Autodesk Inventor part; units mm, degrees
ref_plane "YZ Plane" through (0, 0, 0) normal (1, 0, 0) x (0, 1, 0)
ref_plane "XZ Plane" through (0, 0, 0) normal (0, 1, 0) x (-1, 0, 0)
ref_plane "XY Plane" through (0, 0, 0) normal (0, 0, 1) x (1, 0, 0)
sketch "スケッチ1" plane through (0, 0, 0) normal (0, 1, 0) x (-1, 0, 0)
  circle A0 centre (0, 0) radius 4 construction
  line L0 (0, 0) -> (0, -4.9846) construction
  line L1 (0, 0) -> (4.0815, -2.3565) construction
  line L2 (3.4641, -2) -> (0, -4)
  line L3 (3.4641, 2) -> (3.4641, -2)
  line L4 (0, 4) -> (3.4641, 2)
  line L5 (-3.4641, 2) -> (0, 4)
  line L6 (-3.4641, -2) -> (-3.4641, 2)
  line L7 (0, -4) -> (-3.4641, -2)
  dimension "d0" = 8
  dimension "d1" = 60
  dimension "d4" = 360
extrude "押し出し1" add sketch "スケッチ1" along normal blind 3
fillet "フィレット1" radius 0.5 6 edges at (1.7321, 3, 3) (-1.7321, 3, 3) (-3.4641, 3, 0) (-1.7321, 3, -3) (1.7321, 3, -3) (3.4641, 3, 0)
fillet "フィレット2" radius 0.1 6 edges at (1.7321, 0, 3) (-1.7321, 0, 3) (-3.4641, 0, 0) (-1.7321, 0, -3) (1.7321, 0, -3) (3.4641, 0, 0)
sketch "スケッチ2" plane through (0, 0, 0) normal (0, -1, 0) x (1, 0, 0)
  circle A0 centre (0, 0) radius 2
  dimension "d10" = 4
extrude "押し出し2" add sketch "スケッチ2" along normal blind 12
thread "ねじ1"
sketch "スケッチ3" plane through (0, 3, 0) normal (0, 1, 0) x (1, 0, 0)
  circle A0 centre (0, 0) radius 0.5
  dimension "d15" = 1
extrude "押し出し3" cut sketch "スケッチ3" against normal through all
properties part number "M4×12-VentedHexBolt" material "ステンレス鋼"
Geometry: final body of the model. Coordinates: model frame, mm. A direction names the side the tool comes from. Give positions to 0.01 mm unless a question says otherwise; leave off trailing zeros. Order: outer loops, then holes, each group sorted by start corner. A loop starts at its lowest first (then second) coordinate and runs counter-clockwise, first axis right, second up. Notation, with made-up numbers: (-35.5, 24.25) - (5.5, 24.25) arc R10 cw to (5.5, 33.25) - close; hole circle Ø4 at (-11, 71). An arc over 180 degrees is marked (long way). Use CSV: the item, a comma, the result in double quotes.
1. Mould query, pull axis X, two halves, no side actions, for faces 1 (the face through (-0.108, -4.395, 0.488)), 2 (the face through (-1, 0, -2)), 3 (the face through (-1.69, 2.85, 2.86)). Classes: +X half, -X half, draft (parallel to the pull), parting line (faces both ways), or undercut.
Answers below:
face 1,"undercut"
face 2,"draft"
face 3,"-X half"
2. Section query B-B (y = -5.25). Output: boundary loops of the cut face in (x, z).
Answers below:
outline,"circle Ø4 at (0, 0); hole circle Ø1 at (0, 0)"
3. Section query A-A (z = 0). Output: boundary loops of the cut face in (x, y).
Answers below:
outline,"(-3.46, 0.1) arc R0.1 ccw to (-3.36, 0) - (-2, 0) - (-2, -12) - (-0.5, -12) - (-0.5, 3) - (-2.96, 3) arc R0.5 ccw to (-3.46, 2.5) - close; (0.5, -12) - (2, -12) - (2, 0) - (3.36, 0) arc R0.1 ccw to (3.46, 0.1) - (3.46, 2.5) arc R0.5 ccw to (2.96, 3) - (0.5, 3) - close"
4. Section query C-C (z = -1). Output: boundary loops of the cut face in (x, y), plus the area to 3 significant figures.
Answers below:
outline,"(-3.46, 0.1) arc R0.1 ccw to (-3.36, 0) - (-1.73, 0) - (-1.73, -12) - (1.73, -12) - (1.73, 0) - (3.36, 0) arc R0.1 ccw to (3.46, 0.1) - (3.46, 2.5) arc R0.5 ccw to (2.96, 3) - (-2.96, 3) arc R0.5 ccw to (-3.46, 2.5) - close"
area,"62.2 mm2"
5. Material intervals for line 1 along Z through (x, y) = (0, -0.75); line 2 along Y through (x, z) = (1.5, 2); line 3 along Z through (x, y) = (-0.25, -0.25), sorted ascending. Write a range as from..to.
Answers below:
line 1,"-2..-0.5, 0.5..2"
line 2,"0..3"
line 3,"-1.98..-0.43, 0.43..1.98"
6. Access query for faces 4 (the face through (-1.64, 2.85, -2.89)), 5 (the face through (0, -6, 2)). Directions: +Z, -Z, +X, -X, +Y, -Y. A direction counts if a zero-diameter tool reaches every point of the face in a straight line with its end or side. Return the directions, or none.
Answers below:
face 4,"-Z, -X, +Y"
face 5,"-Y"
7. Contact query for flat-ended pins moving along their axis: pin 1 (4 mm diameter, centred on x = 2, y = -1.5, fed in from +Z); pin 2 (4 mm diameter, centred on x = 0, y = -5, fed in from +Z). Output: stop coordinate, or through.
Answers below:
pin 1,"z = 3.56"
pin 2,"z = 2"
